Geometry: final body of the model. Coordinates: model frame, mm. Give positions to 0.01 mm unless a question says otherwise; leave off trailing zeros. Write each loop counter-clockwise with the first axis right and the second up, starting at its lowest first coordinate (ties: lowest second). Pieces come first, ordered by that corner, then holes. Notation, with made-up numbers: M -35.75,-25 L -25.75,-25 A36 cw -25.75,10 Z; hole C 43.25,-13 d5. An arc over 180 degrees is marked long. Use a Markdown table: item, result. Add a question column.
1) Pin query (flat end, axial travel): pin 1 (0.6 mm diameter, centred on x = -12, y = -1, fed in from -Z); pin 2 (0.6 mm diameter, centred on y = -0.5, z = 15.5, fed in from +X). Return the tip coordinate at first contact, or that it passes through.
2) Section D-D on y = -0.6. State how many separate pieces and enclosed holes the cut face has, then the cut area to 3 significant figures.
3) Section C-C on x = -25.25. Return the cut outline in (y, z), then the cut area to 3 significant figures.
4) Section B-B on x = -11. Return the cut outline in (y, z), then the cut area to 3 significant figures.
5) Section A-A on z = 16.75. Return the cut outline in (x, y), then the cut area to 3 significant figures.
6) Line query: line 1 (X direction, y = -0.4, z = 12.75); line 2 (X direction, y = -0.8, z = 7.5); line 3 (Z direction, x = -15.5, y = -0.55). Output: solid intervals per line, ascending.
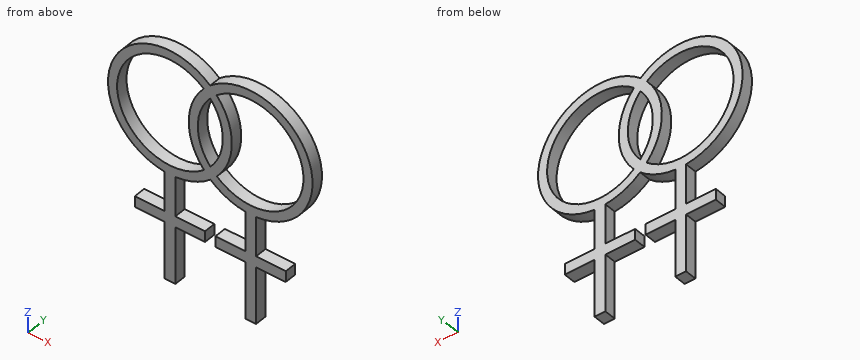
```python
from build123d import *

# Parameters (mm, degrees)
F1_DEPTH = 1.2


with BuildPart() as f1:
    # F0 (on Front) → F1 (new body)
    with BuildSketch(Plane.XZ):
        with BuildLine():
            Line((-22.558661, 13.532754), (-22.558661, 17.550706))
            ThreePointArc((-22.558661, 17.550706), (-20.646676, 18.025718), (-18.973681, 19.066109))
            ThreePointArc((-18.973681, 19.066109), (-17.31198, 18.043084), (-15.41748, 17.575431))
            Line((-15.41748, 17.575431), (-15.41748, 13.55748))
            Line((-15.41748, 13.55748), (-18.455535, 13.55748))
            Line((-18.455535, 13.55748), (-18.455535, 12.45748))
            Line((-18.455535, 12.45748), (-15.41748, 12.45748))
            Line((-15.41748, 12.45748), (-15.41748, 6.657985))
            Line((-15.41748, 6.657985), (-14.31748, 6.657985))
            Line((-14.31748, 6.657985), (-14.31748, 12.45748))
            Line((-14.31748, 12.45748), (-11.279425, 12.45748))
            Line((-11.279425, 12.45748), (-11.279425, 13.55748))
            Line((-11.279425, 13.55748), (-14.31748, 13.55748))
            Line((-14.31748, 13.55748), (-14.31748, 17.575431))
            ThreePointArc((-14.31748, 17.575431), (-9.043176, 26.336733), (-19.002461, 28.658661))
            ThreePointArc((-19.002461, 28.658661), (-28.940326, 26.294523), (-23.658661, 17.550706))
            Line((-23.658661, 17.550706), (-23.658661, 13.532754))
            Line((-23.658661, 13.532754), (-26.696716, 13.532754))
            Line((-26.696716, 13.532754), (-26.696716, 12.432754))
            Line((-26.696716, 12.432754), (-23.658661, 12.432754))
            Line((-23.658661, 12.432754), (-23.658661, 6.63326))
            Line((-23.658661, 6.63326), (-22.558661, 6.63326))
            Line((-22.558661, 6.63326), (-22.558661, 12.432754))
            Line((-22.558661, 12.432754), (-19.520607, 12.432754))
            Line((-19.520607, 12.432754), (-19.520607, 13.532754))
            Line((-19.520607, 13.532754), (-22.558661, 13.532754))
        make_face()
        with BuildLine():
            ThreePointArc((-19.634369, 19.720153), (-28.505536, 23.833831), (-19.659213, 28.000664))
            ThreePointArc((-19.659213, 28.000664), (-21.190733, 23.855777), (-19.634369, 19.720153))
        make_face(mode=Mode.SUBTRACT)
        with BuildLine():
            ThreePointArc((-18.977614, 20.377132), (-20.264355, 23.858556), (-18.998527, 27.347639))
            ThreePointArc((-18.998527, 27.347639), (-17.711786, 23.866214), (-18.977614, 20.377132))
        make_face(mode=Mode.SUBTRACT)
        with BuildLine():
            ThreePointArc((-18.341772, 28.004617), (-9.470605, 23.89094), (-18.316929, 19.724106))
            ThreePointArc((-18.316929, 19.724106), (-16.785408, 23.868994), (-18.341772, 28.004617))
        make_face(mode=Mode.SUBTRACT)
    extrude(amount=F1_DEPTH)


solid = f1.part
```
Found:
| question | item | result |
|---|---|---|
| 1 | pin 1 | z = 12.46 |
| 1 | pin 2 | x = -14.32 |
| 2 | separate pieces | 1 |
| 2 | enclosed holes | 3 |
| 2 | area | 104 mm² |
| 3 | outline | M -1.2,12.43 L 0,12.43 L 0,13.53 L -1.2,13.53 Z; M -1.2,17.9 L 0,17.9 L 0,18.9 L -1.2,18.9 Z; M -1.2,28.8 L 0,28.8 L 0,29.8 L -1.2,29.8 Z |
| 3 | area | 3.71 mm² |
| 4 | outline | M -1.2,18.87 L 0,18.87 L 0,20.11 L -1.2,20.11 Z; M -1.2,27.64 L 0,27.64 L 0,28.88 L -1.2,28.88 Z |
| 4 | area | 2.97 mm² |
| 5 | outline | M -23.66,-1.2 L -22.56,-1.2 L -22.56,0 L -23.66,0 Z; M -15.42,-1.2 L -14.32,-1.2 L -14.32,0 L -15.42,0 Z |
| 5 | area | 2.64 mm² |
| 6 | line 1 | -26.7 to -19.52, -18.46 to -11.28 |
| 6 | line 2 | -23.66 to -22.56, -15.42 to -14.32 |
| 6 | line 3 | 12.46 to 13.56, 17.58 to 18.52, 29.23 to 30.17 |
